from build123d import *

# Parameters (mm, degrees)
F1_DEPTH = 25


with BuildPart() as f1:
    # F0 (on Right) → F1 (new body, symmetric)
    with BuildSketch(Plane.YZ):
        Polygon((-26.998525, 6.460627), (-33.959152, -0.5), (33.959152, -0.5), (0.707107, 32.752045), (18.321796, 50.366735), (17.61469, 51.073841), (-26.291418, 7.167734), (-32.56589, 13.442206), (-33.272997, 12.735099), align=None)
        Polygon((31.544938, 0.5), (-31.544938, 0.5), (0, 32.044938), align=None, mode=Mode.SUBTRACT)
    extrude(amount=F1_DEPTH, both=True)


solid = f1.part
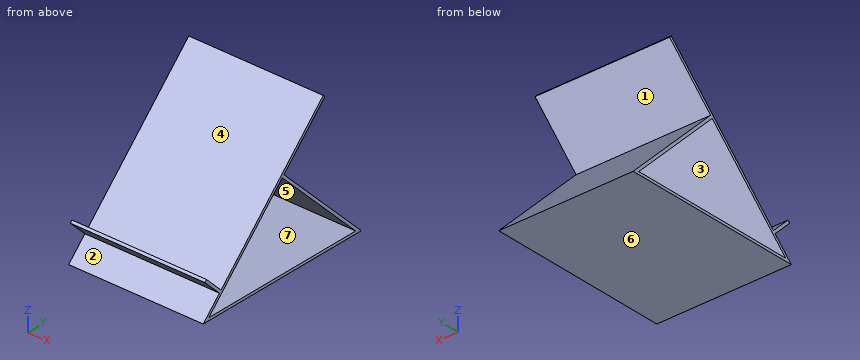
Input: part model. Units: mm. Frame: model coordinates. Face numbers are marked on the shaded views. A direction names the side the tool comes from. Coordinates: 2 decimals unless noted, no trailing zeros. Loops run counter-clockwise (first coordinate to the right, second up) from the corner with the lowest first, then second, coordinate; pieces in that order, holes last.
Q1. Cut plane D-D (z = 5.5). Output: boundary loops of the cut face in (x, y).
Q2. Cut plane A-A (y = -11). Output: boundary loops of the cut face in (x, z).
Q3. Contact query for flat-ended pins moving along their axis: pin 1 (5 mm diameter, centred on x = -11, z = 43.5, fed in from +Y); pin 2 (10 mm diameter, centred on x = 13.5, y = -4, fed in from +Z); pin 3 (1.5 mm diameter, centred on x = 2, z = 23, fed in from +Y); pin 4 (6 mm diameter, centred on y = -25.5, z = 15, fed in from +X). Output: stop coordinate, or through.
Q4. Cut plane C-C (y = 2). Output: boundary loops of the cut face in (x, z).
Q5. Cut plane B-B (x = 8.5). Output: boundary loops of the cut face in (y, z), then the cut area to 3 significant figures.
Q6. Set-up query: the marked faces 1, 2 and 3. Return all of +Z, -Z, +X, -X, +Y, -Y with unobstructed straight access to the full face (end or side cutting, diameter ignored); none if empty.
Q7. Material intervals for line 1 (Z direction, x = 8.5, y = 2); line 2 (Z direction, x = 1.5, y = 11.5); line 3 (Z direction, x = 4, y = -12), sorted ascending.
Q8. Draft query along Z for the marked faces 4, 5, 6 and 7. Return one class per face: +Z half, -Z half, draft (parallel to the pull), parting line (faces both ways), or undercut.
Working result:
1. outline: (-25, -27.96) - (25, -27.96) - (25, -26.54) - (-25, -26.54) - close; (-25, 26.54) - (25, 26.54) - (25, 27.96) - (-25, 27.96) - close
2. outline: (-25, -0.5) - (25, -0.5) - (25, 0.5) - (-25, 0.5) - close; (-25, 21.04) - (25, 21.04) - (25, 22.46) - (-25, 22.46) - close
3. pin 1: stops at y = 13.96
3. pin 2: stops at z = 34.46
3. pin 3: stops at y = 11.21
3. pin 4: passes through
4. outline: (-25, -0.5) - (25, -0.5) - (25, 0.5) - (-25, 0.5) - close; (-25, 30.04) - (25, 30.04) - (25, 31.46) - (-25, 31.46) - close; (-25, 34.04) - (25, 34.04) - (25, 35.46) - (-25, 35.46) - close
5. outline: (-33.96, -0.5) - (33.96, -0.5) - (0.71, 32.75) - (18.32, 50.37) - (17.61, 51.07) - (-26.29, 7.17) - (-32.57, 13.44) - (-33.27, 12.74) - (-27, 6.46) - close; hole (-31.54, 0.5) - (31.54, 0.5) - (0, 32.04) - close
5. area: 192 mm2
6. face 1: +X, -X, +Y
6. face 2: +X, -X, -Y
6. face 3: +X, -X
7. line 1: z = -0.5 to 0.5, 30.04 to 31.46, 34.04 to 35.46
7. line 2: z = -0.5 to 0.5, 20.54 to 21.96, 43.54 to 44.96
7. line 3: z = -0.5 to 0.5, 20.04 to 21.46
8. face 4: +Z half
8. face 5: undercut
8. face 6: -Z half
8. face 7: undercut
